Check sheet for the drawn part. Datum: minimum x, y, z corner. Units: mm. A direction names the side the tool comes from. Give positions to 0.01 mm unless a question says otherwise; leave off trailing zeros. Order: outer loops, then holes, each group sorted by start corner. A loop starts at its lowest first (then second) coordinate and runs counter-clockwise, first axis right, second up. Notation, with made-up numbers: M -24,-3.75 L -2,-3.75 A24 ccw -2,8.25 Z; hole C 12.5,9.5 d5. An arc over 180 degrees is marked long. Answer in a Markdown table with one row per item. Add a question column.
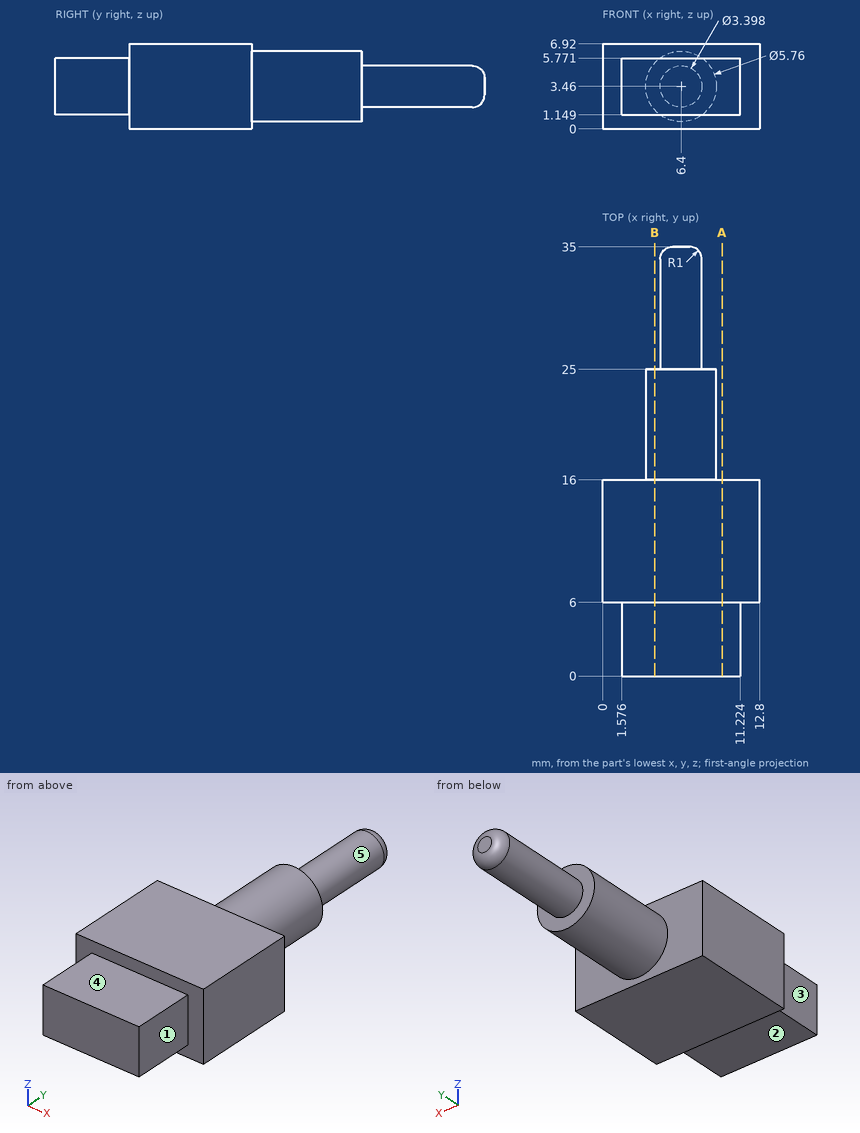
Q1. Tool access check on the marked faces 1, 2, 3, 4 and 5. Record the directions out of +Z, -Z, +X, -X, +Y, -Y that give a thin tool (end or side, any length) a straight path to the whole face; none if there is none.
Q2. Thickness scan on probe 1 along Y at (x, z) = (1.25, 3.25); probe 2 along Z at (x, y) = (6.25, 17); probe 3 along X at (y, z) = (4.5, 2.75) (1 decimal). Record the ranges inside material, lowest first.
Q3. Go/stop test with flat-tipped pins: pin 1 (3 mm diameter, centred on x = 6.5, y = 3.5, fed in from +Z); pin 2 (6.5 mm diameter, centred on x = 7.5, y = 2, fed in from -Z); pin 3 (2.5 mm diameter, centred on y = 4, z = 4.5, fed in from -X). Record where each tip stops, or that it passes through.
Q4. Cross-section at B-B (x = 4.25). Record the boundary of the cut face in (y, z), and give its area (3 significant figures).
Q5. Cross-section at A-A (x = 9.75). Record the boundary of the cut face in (y, z).
Values follow:
| question | item | result |
|---|---|---|
| 1 | face 1 | +Z, -Z, +X, -Y |
| 1 | face 2 | -Z, +X, -X, -Y |
| 1 | face 3 | +Z, -Z, -X, -Y |
| 1 | face 4 | +Z, +X, -X, -Y |
| 1 | face 5 | +Y |
| 2 | probe 1 | 6 to 16 |
| 2 | probe 2 | 0.58 to 6.34 |
| 2 | probe 3 | 1.6 to 11.2 |
| 3 | pin 1 | z = 5.77 |
| 3 | pin 2 | z = 1.15 |
| 3 | pin 3 | x = 1.58 |
| 4 | outline | M 0,1.15 L 6,1.15 L 6,0 L 16,0 L 16,1.54 L 25,1.54 L 25,5.38 L 16,5.38 L 16,6.92 L 6,6.92 L 6,5.77 L 0,5.77 Z |
| 4 | area | 131 mm² |
| 5 | outline | M 0,1.15 L 6,1.15 L 6,0 L 16,0 L 16,6.92 L 6,6.92 L 6,5.77 L 0,5.77 Z |
